```python
from build123d import *

# Parameters (mm, degrees)
ESQUISSE1_R             = 7.5
BOSS_EXTRU_2_DEPTH      = 29
ESQUISSE10_R            = 6
ESQUISSE11_R            = 6
ENL_V_MAT_EXTRU_1_DEPTH = 8
ENL_V_MAT_EXTRU_2_DEPTH = 11.5


with BuildPart() as part:
    # Esquisse1 → Boss.-Extru.2 (new body)
    with BuildSketch(Plane.XY):
        with Locations(Location((-15.770569557, 6.529797245, 0), (0, 0, 180))):
            Circle(ESQUISSE1_R)
    extrude(amount=BOSS_EXTRU_2_DEPTH)

    # Esquisse10 → section 1 of lissage3
    with BuildSketch(Plane.XY.offset(32), mode=Mode.PRIVATE) as lissage3_s1:
        with Locations((-15.770569557, 6.529797245)):
            Circle(ESQUISSE10_R)
    # loft up to a face of the part (lissage3)
    loft([Face(Wire([part.edges().sort_by_distance((-10.636466262, 1.062532539, 29))[0]])), lissage3_s1.sketch])

    # Esquisse11 → Enlèv. mat.-Extru.1 (cut)
    with BuildSketch(Plane(origin=(0, 0, 0), x_dir=(-1, 0, 0), z_dir=(0, 0, -1))):
        with Locations((15.770569557, 6.529797245)):
            Circle(ESQUISSE11_R)
    extrude(amount=-ENL_V_MAT_EXTRU_1_DEPTH, mode=Mode.SUBTRACT)

    # Esquisse13 → Enlèv. mat.-Extru.2 (cut)
    with BuildSketch(Plane.XY.offset(32)):
        Polygon((-15.770569557, 5.107185968), (-18.020569557, 5.107185968), (-18.020569557, 15.896170682), (-13.520569557, 15.896170682), (-13.520569557, 5.107185968), align=None)
    extrude(amount=-ENL_V_MAT_EXTRU_2_DEPTH, mode=Mode.SUBTRACT)


solid = part.part
```
Here's how the part is built. I have some questions about the finished solid (model axes, mm). A direction names the side the tool comes from. Round coordinates to 2 decimals unless told otherwise and drop trailing zeros. Order: outer loops, then holes, each group sorted by start corner. A loop starts at its lowest first (then second) coordinate and runs counter-clockwise, first axis right, second up. Notation, with made-up numbers: (-2.75, 77) -> (18.25, 77) arc R29 ccw to (18.25, 107) -> close; hole circle Ø4 at (-10, 76). An arc over 180 degrees is marked (long way). Use a Markdown table: item, result. Add a question column.
(1) For faces 4 (the face through (-16, 7, 8)), 5 (the face through (-16, 4, 32)), 6 (the face through (-13.521, 9, 26)), which set-ups out of +Z, -Z, +X, -X, +Y, -Y let a thin tool reach every point of the face, with its end or its side?
(2) Suppose I cut it at B-B, the plane z = 18. Please give me the cut outline in (x, y).
(3) I need wall thicknesses on line 1 along Y through (x, z) = (-16, 2.5); line 2 along X through (y, z) = (6.5, 3); line 3 along Z through (x, y) = (-15.5, 10.25). Which ranges of each line are inside material? Lowest first, please.
(4) Suppose I cut it at A-A, the plane z = 28. Please give me the cut outline in (x, y), and give its area (3 significant figures).
(5) For pin 1 Ø2.5 at (x, z) = (-15.5, 25.5) entering from +Y; pin 2 Ø3 at (y, z) = (1, 14) entering from +X; pin 3 Ø4 at (y, z) = (12, 12) entering from +X, each with a flat end and sliding along its axis, tell me the tip position at first contact or that it passes through.
(6) If we mould it in two halves opening along X, with no side actions, what happens to faces 1 (the face through (-19.803, 0.206, 14.297)), 2 (the face through (-16, 5.107, 26)), 3 (the face through (-12, 1, 0))? For each: released by +X, released by -X, zero draft, split by the parting line, or undercut.
Verdict:
| question | item | result |
|---|---|---|
| 1 | face 4 | -Z |
| 1 | face 5 | +Z, +X, -X, +Y, -Y |
| 1 | face 6 | +Z, +Y |
| 2 | outline | circle Ø15 at (-15.77, 6.53) |
| 3 | line 1 | -0.97 to 0.53, 12.53 to 14.03 |
| 3 | line 2 | -23.27 to -21.77, -9.77 to -8.27 |
| 3 | line 3 | 8 to 20.5 |
| 4 | outline | (-18.02, 5.11) -> (-18.02, 13.68) arc R7.5 ccw (long way) to (-13.52, 13.68) -> (-13.52, 5.11) -> close |
| 4 | area | 137 mm2 |
| 5 | pin 1 | y = 5.11 |
| 5 | pin 2 | x = -9.45 |
| 5 | pin 3 | x = -9.12 |
| 6 | face 1 | split by the parting line |
| 6 | face 2 | undercut |
| 6 | face 3 | zero draft |
